Autodesk Inventor part; units mm, degrees
ref_plane "YZ Plane" through (0, 0, 0) normal (1, 0, 0) x (0, 1, 0)
ref_plane "XZ Plane" through (0, 0, 0) normal (0, 1, 0) x (-1, 0, 0)
ref_plane "XY Plane" through (0, 0, 0) normal (0, 0, 1) x (1, 0, 0)
sketch "Sketch1" plane through (0, 0, 0) normal (0, 0, 1) x (1, 0, 0)
  line L0 (0, 0) -> (31.4, 0)
  line L1 (31.4, 0) -> (31.4, 27.4)
  line L2 (31.4, 27.4) -> (0, 27.4)
  line L3 (0, 27.4) -> (0, 0)
  dimension "d0" = 31.4
  dimension "d1" = 27.4
extrude "Extrusion1" add sketch "Sketch1" along normal blind 1
sketch "Sketch17" plane through (0, 0, 1) normal (0, 0, 1) x (1, 0, 0)
  line L0 (2, 25.4) -> (29.4, 25.4) construction
  line L1 (29.4, 25.4) -> (29.4, 2) construction
  line L2 (29.4, 2) -> (2, 2) construction
  line L3 (2, 2) -> (2, 25.4) construction
  line L4 (0, 0) -> (0, 27.4) construction
  line L5 (0, 27.4) -> (31.4, 27.4) construction
  dimension "d169" = 27.4
  dimension "d170" = 23.4
  dimension "d171" = 2
  dimension "d172" = 2
hole "Hole16" at (2, 25.4, 1) at (29.4, 25.4, 1) at (29.4, 2, 1) at (2, 2, 1) direction (0, 0, -1) diameter 2.3 end through all countersink diameter 3.6 countersink angle 90
properties part number "Mixer IQ Box ND20" material "Aluminum-6061"
Can you work these out from the model? Positions are in its coordinate system, mm. Round coordinates to 2 decimals unless told otherwise and drop trailing zeros. Write each loop counter-clockwise with the first axis right and the second up, starting at its lowest first coordinate (ties: lowest second). Pieces come first, ordered by that corner, then holes. Notation, with made-up numbers: (29.25, 13) - (82.25, 13) arc R4 cw to (82.25, 17) - close; hole circle Ø11 at (58.5, 62). An arc over 180 degrees is marked (long way). Write each question's results on one line, items separated by ' | '. Start each with the question number.
1) For pin 1 Ø1.4 at (x, y) = (2, 2) entering from -Z (3 decimals); pin 2 Ø3.5 at (x, y) = (29.4, 2) entering from +Z, each with a flat end and sliding along its axis, tell me the tip position at first contact or that it passes through.
2) Suppose I cut it at A-A (x = 29.4). List the corners of the cut face in (y, z) for me.
3) Suppose I cut it at B-B (y = 25.4). List the corners of the cut face in (x, z) for me.
4) Suppose I cut it at C-C (z = 0.8). List the corners of the cut face in (x, y) for me.
5) Please list where these lines run through material, in increasing order: line 1 (X direction, y = 2, z = 0.15); line 2 (Y direction, x = 29.4, z = 0.1); line 3 (X direction, y = 3, z = 0.85).
6) We'd pull the mould along X, two halves only. Please class faces 1 (the cylindrical face through (1.95, 26.55, 0.17)), 2 (the flat face through (31.4, 13.5, 0.5)), 3 (the flat face through (15, 14, 0)): released by +X, released by -X, zero draft, split by the parting line, or undercut.
Here are the results:
1) pin 1: passes through | pin 2: stops at z = 0.95
2) outline: (0, 0) - (0.85, 0) - (0.85, 0.35) - (0.2, 1) - (0, 1) - close; (3.15, 0) - (24.25, 0) - (24.25, 0.35) - (23.6, 1) - (3.8, 1) - (3.15, 0.35) - close; (26.55, 0) - (27.4, 0) - (27.4, 1) - (27.2, 1) - (26.55, 0.35) - close
3) outline: (0, 0) - (0.85, 0) - (0.85, 0.35) - (0.2, 1) - (0, 1) - close; (3.15, 0) - (28.25, 0) - (28.25, 0.35) - (27.6, 1) - (3.8, 1) - (3.15, 0.35) - close; (30.55, 0) - (31.4, 0) - (31.4, 1) - (31.2, 1) - (30.55, 0.35) - close
4) outline: (0, 0) - (31.4, 0) - (31.4, 27.4) - (0, 27.4) - close; hole circle Ø3.2 at (2, 2); hole circle Ø3.2 at (2, 25.4); hole circle Ø3.2 at (29.4, 2); hole circle Ø3.2 at (29.4, 25.4)
5) line 1: x = 0 to 0.85, 3.15 to 28.25, 30.55 to 31.4 | line 2: y = 0 to 0.85, 3.15 to 24.25, 26.55 to 27.4 | line 3: x = 0 to 0.69, 3.31 to 28.09, 30.71 to 31.4
6) face 1: undercut | face 2: released by +X | face 3: zero draft
